```python
from build123d import *

# Parameters (mm, degrees)
F0_W     = 25.4
F0_H     = 44.45
F1_DEPTH = 57.15
F3_DEPTH = 12.7
F5_DEPTH = 25.4


with BuildPart() as f1:
    # F0 (on Right) → F1 (new body)
    with BuildSketch(Plane.YZ):
        with Locations((12.7, 22.225)):
            Rectangle(F0_W, F0_H)
    extrude(amount=F1_DEPTH)

    # F2 (on face) → F3 (cut)
    with BuildSketch(Plane.XZ):
        Polygon((57.15, 44.45), (19.05, 44.45), (44.45, 0), (57.15, 0), align=None)
    extrude(amount=-F3_DEPTH, mode=Mode.SUBTRACT)

    # F4 (on face) → F5 (cut)
    with BuildSketch(Plane.XZ):
        with BuildLine():
            ThreePointArc((38.050965, 11.198312), (42.734358, 15.850529), (44.45, 22.225))
            ThreePointArc((44.45, 22.225), (38.124471, 33.209358), (25.449035, 33.251688))
            Line((25.449035, 33.251688), (38.050965, 11.198312))
        make_face()
        with BuildLine():
            Line((38.050965, 11.198312), (25.449035, 33.251688))
            ThreePointArc((25.449035, 33.251688), (20.723312, 15.924035), (38.050965, 11.198312))
        make_face()
    extrude(amount=-F5_DEPTH, mode=Mode.SUBTRACT)


solid = f1.part
```
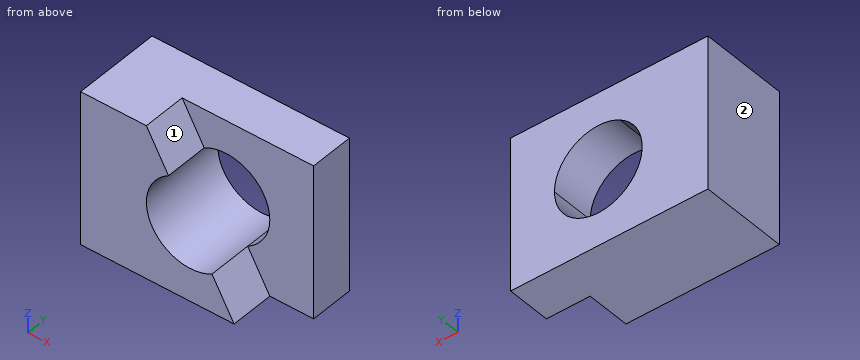
The listing builds one solid part. Answer for the finished solid, in the listing's coordinates (mm). Face numbers are marked on the shaded views. A direction names the side the tool comes from. Round coordinates to 2 decimals unless told otherwise and drop trailing zeros. Write each loop counter-clockwise with the first axis right and the second up, starting at its lowest first coordinate (ties: lowest second). Pieces come first, ordered by that corner, then holes. Notation, with made-up numbers: (77, -39.5) -> (114, -39.5) arc R12 ccw to (114, -27.5) -> close; hole circle Ø9 at (-9, -39). An arc over 180 degrees is marked (long way). Answer as a JSON object with one key per item and string values. Group by question number.
Q1. Section C-C (y = 2) is taken. Write down the section's boundary in (x, z) (3 decimals).
Q2. Straight lines are drawn through the part: line 1 along X through (y, z) = (21, 22.5); line 2 along Y through (x, z) = (48, 12); line 3 along Z through (x, y) = (39.5, 16.25). For each, find the intervals that lie inside material, in ascending order.
Q3. Which of the six approach directions +Z, -Z, +X, -X, +Y, -Y give full straight-line access (tool end or side, diameter ignored) to the marked faces 1 and 2?
Q4. Section D-D (z = 26) is taken. Write down the section's boundary in (x, y).
Q5. Section A-A (x = 31.75) is taken. Write down the section's boundary in (y, z) (3 decimals), plus the area to 3 significant figures.
Q6. Section B-B (y = 23.5) is taken. Write down the section's boundary in (x, z) (3 decimals), plus the area to 3 significant figures.
Check values:
{
 "1": {"outline": "(0, 0) -> (44.45, 0) -> (38.051, 11.198) arc R12.7 cw to (25.449, 33.252) -> (19.05, 44.45) -> (0, 44.45) -> close"},
 "2": {"line 1": "0 to 19.05, 44.45 to 57.15", "line 2": "12.7 to 25.4", "line 3": "0 to 12.16, 32.29 to 44.45"},
 "3": {"face 1": "+Z, +X, -Y", "face 2": "+Z, -Z, -X, +Y, -Y"},
 "4": {"outline": "(0, 0) -> (19.62, 0) -> (19.62, 25.4) -> (0, 25.4) -> close; (43.88, 12.7) -> (57.15, 12.7) -> (57.15, 25.4) -> (43.88, 25.4) -> close"},
 "5": {"outline": "(0, 0) -> (25.4, 0) -> (25.4, 9.525) -> (0, 9.525) -> close; (12.7, 34.925) -> (25.4, 34.925) -> (25.4, 44.45) -> (12.7, 44.45) -> close", "area": "363 mm^2"},
 "6": {"outline": "(0, 0) -> (57.15, 0) -> (57.15, 44.45) -> (0, 44.45) -> close; hole circle Ø25.4 at (31.75, 22.225)", "area": "2,030 mm^2"}
}
